The model under review builds one solid part; all positions refer to its coordinate system, in mm. Give positions to 0.01 mm unless a question says otherwise; leave off trailing zeros. Loops run counter-clockwise (first coordinate to the right, second up) from the corner with the lowest first, then second, coordinate; pieces in that order, holes last. Notation, with made-up numbers: M 58,71.5 L 77,71.5 A29 cw 77,106.5 Z; hole C 79.5,28.25 d1. An arc over 180 degrees is marked long. Return JSON: item names as keys, results as strings.
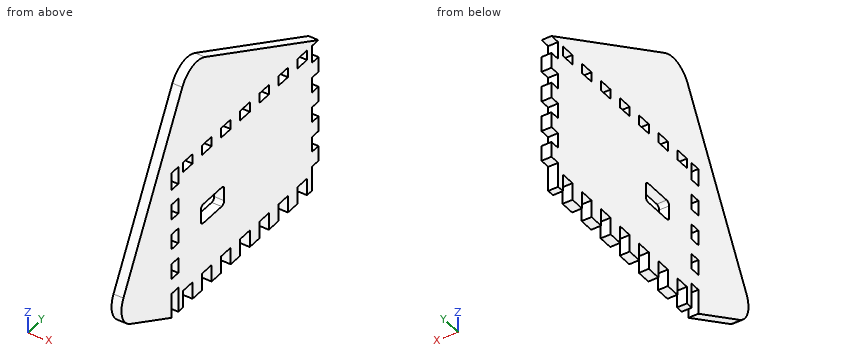
```python
from build123d import *

# Parameters (mm, degrees)
SCHIZZO1_W                    = 50
SCHIZZO1_H                    = 80
ESTRUSIONE_ESTRUSIONE1_DEPTH  = 4
SCHIZZO2_W                    = 4
SCHIZZO2_H                    = 2.857142857
SCHIZZO2_W_2                  = 7
ESTRUSIONE_ESTRUSIONE2_DEPTH  = 4
SCHIZZO3_W                    = 4
SCHIZZO3_H                    = 5.714285715
SCHIZZO3_W_2                  = 7
ESTRUSIONE_ESTRUSIONE3_DEPTH  = 4
RIPETIZIONE_A_L1_COUNT        = 6
RIPETIZIONE_A_L1_PITCH        = 11.428571
SCHIZZO4_W                    = 6.25
SCHIZZO4_H                    = 4
ESTRUSIONE_ESTRUSIONE4_DEPTH  = 4
RIPETIZIONE_A_L2_COUNT        = 4
RIPETIZIONE_A_L2_PITCH        = 12.5
ESTRUSIONE_ESTRUSIONE5_DEPTH  = 4
RACCORDO1_R                   = 10
TAGLIO_ESTRUSIONE1_DEPTH      = 102.592322545
TAGLIO_ESTRUSIONE1_DEPTH_BACK = 102.592322545


with BuildPart() as part:
    # Schizzo1 → Estrusione-Estrusione1 (new body)
    with BuildSketch(Plane(origin=(0, 0, 0), x_dir=(0, 0, -1), z_dir=(1, 0, 0))):
        with Locations((25, 40)):
            Rectangle(SCHIZZO1_W, SCHIZZO1_H)
    extrude(amount=ESTRUSIONE_ESTRUSIONE1_DEPTH)

    # Schizzo2 → Estrusione-Estrusione2 (add)
    with BuildSketch(Plane(origin=(4, 0, 0), x_dir=(0, 0, -1), z_dir=(1, 0, 0))):
        with Locations((-2, 78.571428572)):
            Rectangle(SCHIZZO2_W, SCHIZZO2_H)
        with Locations((53.5, 78.571428572)):
            Rectangle(SCHIZZO2_W_2, SCHIZZO2_H)
        with Locations((53.5, 1.428571429)):
            Rectangle(SCHIZZO2_W_2, SCHIZZO2_H)
        with Locations((-2, 1.428571429)):
            Rectangle(SCHIZZO2_W, SCHIZZO2_H)
    extrude(amount=-ESTRUSIONE_ESTRUSIONE2_DEPTH)

    # Schizzo3 → Estrusione-Estrusione3 (add)
    with BuildSketch(Plane(origin=(4, 0, 0), x_dir=(0, 0, -1), z_dir=(1, 0, 0))):
        with Locations((-2, 68.571428572)):
            Rectangle(SCHIZZO3_W, SCHIZZO3_H)
        with Locations((53.5, 68.571428572)):
            Rectangle(SCHIZZO3_W_2, SCHIZZO3_H)
    estrusione_estrusione3 = extrude(amount=-ESTRUSIONE_ESTRUSIONE3_DEPTH)

    # Ripetizione a L1: Estrusione-Estrusione3 ×6
    with Locations(*[(0, -i * RIPETIZIONE_A_L1_PITCH, 0) for i in range(1, RIPETIZIONE_A_L1_COUNT)]):
        add(estrusione_estrusione3)

    # Schizzo4 → Estrusione-Estrusione4 (add)
    with BuildSketch(Plane(origin=(4, 0, 0), x_dir=(0, 0, -1), z_dir=(1, 0, 0))):
        with Locations((6.25, 82)):
            Rectangle(SCHIZZO4_W, SCHIZZO4_H)
        with Locations((6.25, -2)):
            Rectangle(SCHIZZO4_W, SCHIZZO4_H)
    estrusione_estrusione4 = extrude(amount=-ESTRUSIONE_ESTRUSIONE4_DEPTH)

    # Ripetizione a L2: Estrusione-Estrusione4 ×4
    with Locations(*[(0, 0, -i * RIPETIZIONE_A_L2_PITCH) for i in range(1, RIPETIZIONE_A_L2_COUNT)]):
        add(estrusione_estrusione4)

    # Schizzo5 → Estrusione-Estrusione5 (add)
    with BuildSketch(Plane(origin=(4, 0, 0), x_dir=(0, 0, -1), z_dir=(1, 0, 0))):
        Polygon((46.875, -4), (57, -4), (39.160080614, -37.552008529), (-44.872956134, 7.129149682), (-4, 84), (-4, 80), (-4, -4), align=None)
    extrude(amount=-ESTRUSIONE_ESTRUSIONE5_DEPTH)

    # Raccordo1
    raccordo1_edges = [part.edges().sort_by_distance(p)[0] for p in [
        (2, -37.552008529, -39.160080614),
        (2, 7.129149682, 44.872956134),
    ]]
    fillet(raccordo1_edges, radius=RACCORDO1_R)

    # Schizzo6 → Taglio-Estrusione1 (cut, two sides: drawn at the far end of the back side and taken through both)
    with BuildSketch(Plane(origin=(4, 0, 0), x_dir=(0, 0, -1), z_dir=(1, 0, 0)).offset(-TAGLIO_ESTRUSIONE1_DEPTH_BACK)):
        with BuildLine():
            Line((21.2, 26), (21.2, 15))
            ThreePointArc((21.2, 15), (21.639339828, 13.939339828), (22.7, 13.5))
            Line((22.7, 13.5), (27.7, 13.5))
            ThreePointArc((27.7, 13.5), (28.760660172, 13.939339828), (29.2, 15))
            Line((29.2, 15), (29.2, 26))
            ThreePointArc((29.2, 26), (28.760660172, 27.060660172), (27.7, 27.5))
            Line((27.7, 27.5), (22.7, 27.5))
            ThreePointArc((22.7, 27.5), (21.639339828, 27.060660172), (21.2, 26))
        make_face()
    extrude(amount=TAGLIO_ESTRUSIONE1_DEPTH + TAGLIO_ESTRUSIONE1_DEPTH_BACK, mode=Mode.SUBTRACT)


solid = part.part
```
1) Insertion check: pin 1 (2 mm diameter, centred on x = 1.5, y = 81.5, fed in from -Z) (3 decimals); pin 2 (2 mm diameter, centred on x = 3, z = 2, fed in from -Y); pin 3 (1.2 mm diameter, centred on x = 1, y = 18.5, fed in from -Z). Each pin has a flat end and moves straight along its axis. Give the tip position at first contact, or say it passes through.
From the geometry:
{"pin 1": "z = -46.875", "pin 2": "y = -16.2", "pin 3": "z = -50"}
2) Consider section C-C on z = -24. Write out the cut boundary in (x, y), then the cut area to 3 significant figures.
From the geometry:
{"outline": "M 0,-29.49 L 4,-29.49 L 4,-4 L 0,-4 Z; M 0,0 L 4,0 L 4,13.5 L 0,13.5 Z; M 0,27.5 L 4,27.5 L 4,80 L 0,80 Z", "area": "366 mm²"}
3) Consider section D-D on x = 3.25. Count the separate pieces of the cut face and the enclosed holes in it, then the cut area to 3 significant figures.
From the geometry:
{"separate pieces": "1", "enclosed holes": "12", "area": "7,750 mm²"}
4) Wall thickness on L1, parallel to Y at x = 2.6, z = -25; L2, parallel to Z at x = 3.7, y = 15; L3, parallel to Y at x = 2.8, z = -28: over which ranges is each line inside the solid? List them lowest first. Write a range as from..to.
From the geometry:
{"L1": "-30.02..-4, 0..13.5, 27.5..80", "L2": "-50..-29.2, -21.2..0, 4..40.62", "L3": "-31.62..-4, 0..13.53, 27.47..80"}
5) Consider section A-A on z = -13. Write out the cut boundary in (x, y).
From the geometry:
{"outline": "M 0,-23.64 L 4,-23.64 L 4,-4 L 0,-4 Z; M 0,0 L 4,0 L 4,80 L 0,80 Z"}
6) Consider section B-B on y = 51.5. Write out the cut boundary in (x, z), then the cut area to 3 significant figures.
From the geometry:
{"outline": "M 0,-50 L 4,-50 L 4,0 L 0,0 Z; M 0,4 L 4,4 L 4,21.28 L 0,21.28 Z", "area": "269 mm²"}
